Study the drawing (mm; zero at the part's minimum x, y, z) and answer. Give positions to 0.01 mm unless a question says otherwise; leave off trailing zeros. Order: outer loops, then holes, each group sorted by start corner. A loop starts at its lowest first (then second) coordinate and runs counter-clockwise, first axis right, second up. Notation, with made-up numbers: (11.5, 14.25) - (32.5, 14.25) arc R12 cw to (32.5, 34.25) - close; hole circle Ø10 at (20.5, 40.25). An arc over 180 degrees is marked (long way). Use CSV: the item, a comma, the result in double quotes.
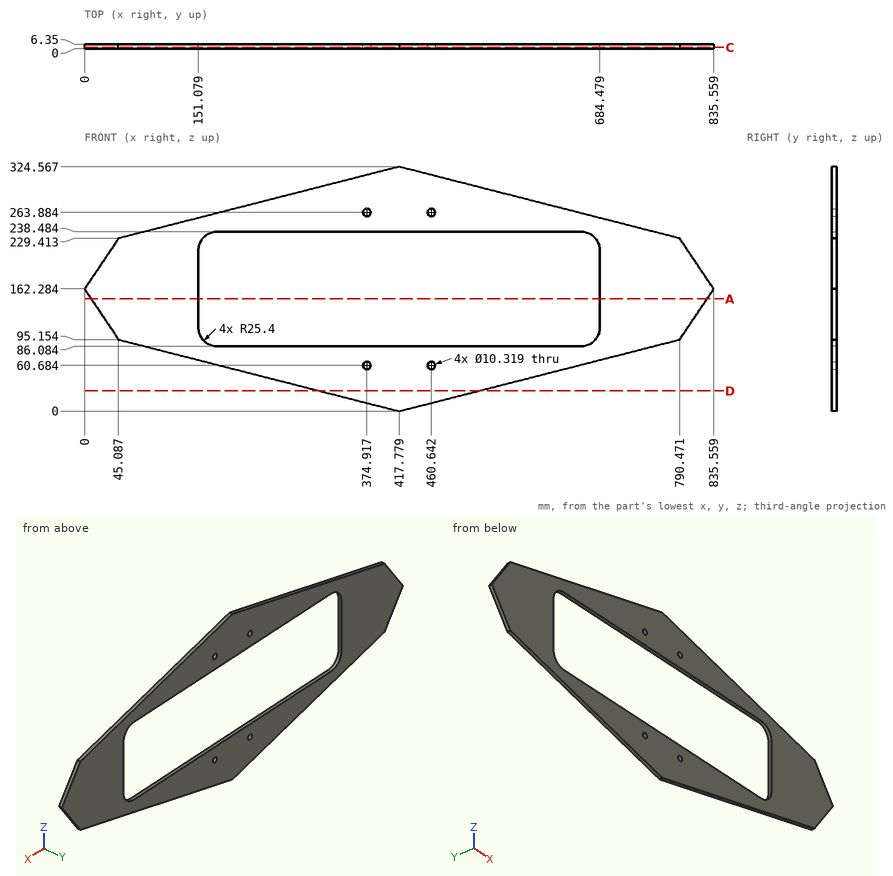
Item 1: Find the intervals of material crossed by line 1 along Z through (x, y) = (484.5, 3) (1 decimal); line 2 along Z through (x, y) = (442.5, 1) (1 decimal); line 3 along X through (y, z) = (2, 142.5), in increasing order.
Taken from the geometry:
line 1,"17 to 86.1, 238.5 to 307.5"
line 2,"6.3 to 86.1, 238.5 to 318.3"
line 3,"13.29 to 151.08, 684.48 to 822.27"
Item 2: The part is cut by section C-C (y = 1.75). Give the vertices of the cut face in (x, z) (1 decimal), and give its area (3 significant figures).
Taken from the geometry:
outline,"(0, 162.3) - (45.1, 95.2) - (417.8, 0) - (790.5, 95.2) - (835.6, 162.3) - (790.5, 229.4) - (417.8, 324.6) - (45.1, 229.4) - close; hole (151.1, 111.5) arc R25.4 ccw to (176.5, 86.1) - (659.1, 86.1) arc R25.4 ccw to (684.5, 111.5) - (684.5, 213.1) arc R25.4 ccw to (659.1, 238.5) - (176.5, 238.5) arc R25.4 ccw to (151.1, 213.1) - close; hole circle Ø10.3 at (374.9, 60.7); hole circle Ø10.3 at (374.9, 263.9); hole circle Ø10.3 at (460.6, 60.7); hole circle Ø10.3 at (460.6, 263.9)"
area,"96,000 mm^2"
Item 3: The part is cut by section A-A (z = 149). Give the vertices of the cut face in (x, y).
Taken from the geometry:
outline,"(8.92, 0) - (151.08, 0) - (151.08, 6.35) - (8.92, 6.35) - close; (684.48, 0) - (826.64, 0) - (826.64, 6.35) - (684.48, 6.35) - close"
Item 4: Each of these flat-tipped pins is pushed along its axis until it touches: pin 1 (9.5 mm diameter, centred on x = 460.64, z = 60.68, fed in from +Y) (3 decimals); pin 2 (3 mm diameter, centred on y = 3, z = 185.5, fed in from +X); pin 3 (3 mm diameter, centred on y = 2, z = 137.5, fed in from -X). Where does it stop, or does it pass through?
Taken from the geometry:
pin 1,"through"
pin 2,"x = 820.97"
pin 3,"x = 15.64"
Item 5: The part is cut by section D-D (z = 27). Give the vertices of the cut face in (x, y), and give its area (3 significant figures).
Taken from the geometry:
outline,"(312.03, 0) - (523.53, 0) - (523.53, 6.35) - (312.03, 6.35) - close"
area,"1,340 mm^2"
